from build123d import *

# Parameters (mm, degrees)
CROQUIS1_R                 = 6
SALIENTE_EXTRUIR1_DEPTH    = 65
CORTAR_EXTRUIR1_DEPTH      = 148.783471464
CORTAR_EXTRUIR1_DEPTH_BACK = 148.783471464
CROQUIS2_W                 = 59
CROQUIS2_H                 = 249
CROQUIS3_R                 = 6
SALIENTE_EXTRUIR2_DEPTH    = 65


with BuildPart() as part:
    # Croquis1 → Saliente-Extruir1 (new body)
    with BuildSketch(Plane.XY):
        with BuildLine():
            Line((-74.262739229, 110), (-20.262739229, 110))
            ThreePointArc((-20.262739229, 110), (-17.790684157, 54.650853089), (11.872762465, 7.856419076))
            ThreePointArc((11.872762465, 7.856419076), (12.856419076, -16.872762465), (-11.872762465, -17.856419076))
            ThreePointArc((-11.872762465, -17.856419076), (-55.070234136, 40.214949961), (-74.262739229, 110))
        make_face()
        with Locations((0, -5)):
            Circle(CROQUIS1_R, mode=Mode.SUBTRACT)
    extrude(amount=SALIENTE_EXTRUIR1_DEPTH)

    # Croquis2 → Cortar-Extruir1 (cut, two sides: drawn at the far end of the back side and taken through both)
    with BuildSketch(Plane(origin=(0, 0, 0), x_dir=(0, 0, -1), z_dir=(1, 0, 0)).offset(-CORTAR_EXTRUIR1_DEPTH_BACK)):
        with Locations((-32.5, -22.5)):
            Rectangle(CROQUIS2_W, CROQUIS2_H)
    extrude(amount=CORTAR_EXTRUIR1_DEPTH + CORTAR_EXTRUIR1_DEPTH_BACK, mode=Mode.SUBTRACT)

    # Croquis3 → Saliente-Extruir2 (add)
    with BuildSketch(Plane(origin=(0, 110, 0), x_dir=(1, 0, 0), z_dir=(0, 1, 0))):
        with Locations((-47.262739229, -31.234778604)):
            Circle(CROQUIS3_R)
    extrude(amount=SALIENTE_EXTRUIR2_DEPTH)


solid = part.part
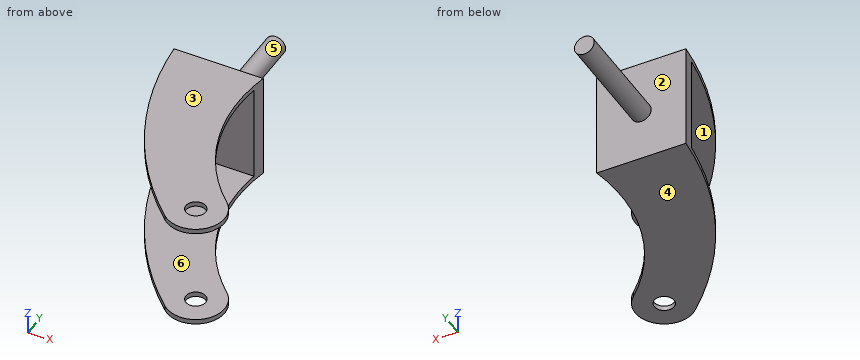
Input: part model. Units: mm. Frame: model coordinates. Face numbers are marked on the shaded views. A direction names the side the tool comes from. Give positions to 0.01 mm unless a question says otherwise; leave off trailing zeros. Loops run counter-clockwise (first coordinate to the right, second up) from the corner with the lowest first, then second, coordinate; pieces in that order, holes last. Notation, with made-up numbers: (54.5, 5) -> (81.5, 5) arc R25 ccw to (81.5, 35) -> close; hole circle Ø1 at (-37, -19). An arc over 180 degrees is marked (long way). Answer as a JSON object with one key per item and string values. Group by question number.
Item 1: Pull-direction query (Z, two-part tool) for the marked faces 1, 2 and 3; classes: released by +Z, released by -Z, zero draft, split by the parting line, or undercut.
Item 2: Pin query (flat end, axial travel): P1, Ø3, axis at y = 119.5, z = 34.5, coming from the -X side; P2, Ø2, axis at x = -64.5, z = 51, coming from the -Y side. Return the tip coordinate at first contact, or that it passes through.
Item 3: Reachability of the marked faces 4, 5 and 6 from +Z, -Z, +X, -X, +Y, -Y: full face, straight path, thin tool, end or side. Return the list, or none.
Item 4: Cut plane D-D, the plane z = 28. Return the cut outline in (x, y).
Item 5: Cut plane B-B, the plane y = -5. Return the cut outline in (x, z), and give its area (3 significant figures).
Item 6: Cut plane C-C, the plane x = -2.5. Return the cut outline in (y, z).
Item 7: Line query: probe 1 along Z at (x, y) = (-17, 6); probe 2 along Y at (x, z) = (-48, 25.5); probe 3 along X at (y, z) = (-5, 63). Output: solid intervals per line, ascending.
Item 8: Cut plane A-A, the plane y = 25.5. Return the cut outline in (x, z).
Checks:
{
 "1": {"face 1": "undercut", "face 2": "zero draft", "face 3": "released by +Z"},
 "2": {"P1": "stops at x = -53", "P2": "stops at y = 102"},
 "3": {"face 4": "-Z, +X, -X, +Y, -Y", "face 5": "+Y", "face 6": "+X, -X, -Y"},
 "4": {"outline": "(-74.26, 110) arc R196.11 ccw to (-73.43, 102) -> (-21.7, 102) arc R107.69 cw to (-20.26, 110) -> (-42.21, 110) -> (-42.21, 175) -> (-52.32, 175) -> (-52.32, 110) -> close"},
 "5": {"outline": "(-24.57, 0) -> (-6, 0) -> (-6, 3) -> (-24.57, 3) -> close; (-24.57, 62) -> (-6, 62) -> (-6, 65) -> (-24.57, 65) -> close; (6, 0) -> (17.5, 0) -> (17.5, 3) -> (6, 3) -> close; (6, 62) -> (17.5, 62) -> (17.5, 65) -> (6, 65) -> close", "area": "180 mm²"},
 "6": {"outline": "(-22.32, 0) -> (-10.45, 0) -> (-10.45, 3) -> (-22.32, 3) -> close; (-22.32, 62) -> (-10.45, 62) -> (-10.45, 65) -> (-22.32, 65) -> close; (0.45, 0) -> (24.1, 0) -> (24.1, 3) -> (0.45, 3) -> close; (0.45, 62) -> (24.1, 62) -> (24.1, 65) -> (0.45, 65) -> close"},
 "7": {"probe 1": "z = 0 to 3, 62 to 65", "probe 2": "y = 102 to 175", "probe 3": "x = -24.57 to -6, 6 to 17.5"},
 "8": {"outline": "(-47.1, 0) -> (-3.49, 0) -> (-3.49, 3) -> (-47.1, 3) -> close; (-47.1, 62) -> (-3.49, 62) -> (-3.49, 65) -> (-47.1, 65) -> close"}
}
